Model file for the job. Use its own axes, mm. A direction names the side the tool comes from. Give positions to 0.01 mm unless a question says otherwise; leave off trailing zeros. Write each loop counter-clockwise with the first axis right and the second up, starting at its lowest first coordinate (ties: lowest second). Pieces come first, ordered by that corner, then holes.
```python
from build123d import *

# Parameters (mm, degrees)
SKETCH1_W               = 80
SKETCH1_H               = 57.5
BOSS_EXTRUDE1_DEPTH     = 8
BOSS_EXTRUDE2_START     = -10
SKETCH3_R               = 3.1
BOSS_EXTRUDE2_DEPTH     = 5
CUT_EXTRUDE1_DEPTH      = 10
CUT_EXTRUDE1_DEPTH_BACK = 63
MOVE_FACE1_BY           = 6
SKETCH5_W               = 80
SKETCH5_H               = 79.999909439
BOSS_EXTRUDE3_DEPTH     = 2
FILLET1_R               = 2
SKETCH6_R               = 2.275
CUT_EXTRUDE2_DEPTH      = 2
SKETCH7_W               = 58.936081431
SKETCH7_H               = 58.936081431
CUT_EXTRUDE3_DEPTH      = 2
FILLET2_R               = 4


with BuildPart() as part:
    # Sketch1 → Boss-Extrude1 (new body)
    with BuildSketch(Plane(origin=(0, 1.4, 0), x_dir=(1, 0, 0), z_dir=(0, 1, 0))):
        with Locations((0, 12.22)):
            Rectangle(SKETCH1_W, SKETCH1_H)
    extrude(amount=BOSS_EXTRUDE1_DEPTH)

    # Sketch3 → Boss-Extrude2 (add)
    # profile 1 of 2: a face of its own
    with BuildSketch(Plane(origin=(0, 0, -36.97), x_dir=(-1, 0, 0), z_dir=(0, 0, -1)).offset(BOSS_EXTRUDE2_START)):
        with BuildLine():
            Line((-30, 1.4), (-40, 1.4))
            Line((-40, 1.4), (-34.195661174, -6.999383953))
            ThreePointArc((-34.195661174, -6.999383953), (-26.018142719, -7.286661669), (-28.090628592, 0.629090909))
            Line((-28.090628592, 0.629090909), (-30, 1.4))
        make_face()
        with Locations(Location((-30, -4.1, 0), (0, 0, 180))):
            Circle(SKETCH3_R, mode=Mode.SUBTRACT)
    # profile 2 of 2: a face of its own
    with BuildSketch(Plane(origin=(0, 0, -36.97), x_dir=(-1, 0, 0), z_dir=(0, 0, -1)).offset(BOSS_EXTRUDE2_START)):
        with BuildLine():
            Line((34.195661174, -6.999383953), (40, 1.4))
            Line((40, 1.4), (30, 1.4))
            Line((30, 1.4), (28.090628592, 0.629090909))
            ThreePointArc((28.090628592, 0.629090909), (26.018142719, -7.286661669), (34.195661174, -6.999383953))
        make_face()
        with Locations(Location((30, -4.1, 0), (0, 0, 180))):
            Circle(SKETCH3_R, mode=Mode.SUBTRACT)
    boss_extrude2 = extrude(amount=-BOSS_EXTRUDE2_DEPTH)

    # Mirror1: Boss-Extrude2 across plane
    add(boss_extrude2.mirror(Plane.XY.offset(-13.22)))

    # Sketch4 → Cut-Extrude1 (cut, two sides: drawn at the far end of the back side and taken through both)
    with BuildSketch(Plane(origin=(0, 0, -21.97), x_dir=(-1, 0, 0), z_dir=(0, 0, -1)).offset(-CUT_EXTRUDE1_DEPTH_BACK)):
        Polygon((-30, -4.1), (-20, -9.873502692), (-40, -9.873502692), align=None)
        Polygon((20, -9.873502692), (40, -9.873502692), (30, -4.1), align=None)
    extrude(amount=CUT_EXTRUDE1_DEPTH + CUT_EXTRUDE1_DEPTH_BACK, mode=Mode.SUBTRACT)

    # Move Face1: a face moved inward by 6.0
    extrude(part.faces().sort_by_distance((0, 9.4, -12.22))[0], amount=MOVE_FACE1_BY, dir=(0, -1, 0), mode=Mode.SUBTRACT)

    # Sketch5 → Boss-Extrude3 (add)
    with BuildSketch(Plane(origin=(0, 3.4, 0), x_dir=(1, 0, 0), z_dir=(0, 1, 0))):
        with Locations((0, 23.46995472)):
            Rectangle(SKETCH5_W, SKETCH5_H)
    extrude(amount=-BOSS_EXTRUDE3_DEPTH)

    # Fillet1
    fillet1_edges = [part.edges().sort_by_distance(p)[0] for p in [
        (40, 2.4, -63.469909439),
        (-40, 2.4, -63.469909439),
        (40, 2.4, 16.53),
        (-40, 2.4, 16.53),
    ]]
    fillet(fillet1_edges, radius=FILLET1_R)

    # Sketch6 → Cut-Extrude2 (cut)
    with BuildSketch(Plane(origin=(0, 3.4, 0), x_dir=(1, 0, 0), z_dir=(0, 1, 0))):
        with Locations(Location((35.75, 59.219909439, 0), (0, 0, 180))):
            Circle(SKETCH6_R)
        with Locations(Location((35.75, -12.280045281, 0), (0, 0, 180))):
            Circle(SKETCH6_R)
        with Locations(Location((-35.74995472, 59.219909439, 0), (0, 0, 180))):
            Circle(SKETCH6_R)
        with Locations(Location((-35.74995472, -12.280045281, 0), (0, 0, 180))):
            Circle(SKETCH6_R)
    extrude(amount=-CUT_EXTRUDE2_DEPTH, mode=Mode.SUBTRACT)

    # Sketch7 → Cut-Extrude3 (cut)
    with BuildSketch(Plane(origin=(0, 3.4, 0), x_dir=(1, 0, 0), z_dir=(0, 1, 0))):
        with Locations((2.264e-05, 23.469932079)):
            Rectangle(SKETCH7_W, SKETCH7_H)
    extrude(amount=-CUT_EXTRUDE3_DEPTH, mode=Mode.SUBTRACT)

    # Fillet2
    fillet2_edges = [part.edges().sort_by_distance(p)[0] for p in [
        (29.468063356, 2.4, -52.937972794),
        (29.468063356, 2.4, 5.998108637),
        (-29.468018075, 2.4, 5.998108637),
        (-29.468018075, 2.4, -52.937972794),
    ]]
    fillet(fillet2_edges, radius=FILLET2_R)


solid = part.part
```
1. Which spindle directions (+Z, -Z, +X, -X, +Y, -Y) get a long thin tool onto all of the face, cutting with end or side? Do faces 5 (the flat face through (33, -2, -26.97)), 6 (the flat face through (-26.461, -6.143, -1.935)), 7 (the flat face through (33, -2, 0.53)), 8 (the cylindrical face through (25.159, -2.497, -24.505)). Say none if no direction does.
Calculated:
face 5: -Z, +X, -X, -Y
face 6: +Z, -Z, -Y
face 7: +Z, +X, -X, -Y
face 8: +Z, -Z
2. Slice it at C-C, the plane y = -2.25. State how many separate pieces and enclosed holes the cut face has, and give its area (3 significant figures).
Calculated:
separate pieces: 8
enclosed holes: 0
area: 145 mm2
3. Probe probe 1 along Z at (x, y) = (35.75, 2.55); probe 2 along X at (y, z) = (2.75, -59.5); probe 3 along X at (y, z) = (1.5, 2). List the from-to ranges inside material, lowest first.
Calculated:
probe 1: z = -63.47 to -61.49, -56.94 to 10.01, 14.56 to 16.53
probe 2: x = -40 to -38.01, -33.49 to 33.49, 38.01 to 40
probe 3: x = -40 to -29.47, 29.47 to 40
4. Slice it at B-B, the plane x = -4. Write the cut outline in (y, z).
Calculated:
outline: (1.4, -63.47) - (3.4, -63.47) - (3.4, -52.94) - (1.4, -52.94) - close; (1.4, 6) - (3.4, 6) - (3.4, 16.53) - (1.4, 16.53) - close
5. Slice it at D-D, the plane x = 35.75. Write the cut outline in (y, z), and give its area (3 significant figures).
Calculated:
outline: (-4.75, -26.97) - (1.4, -26.97) - (1.4, -56.94) - (3.4, -56.94) - (3.4, 10.01) - (1.4, 10.01) - (1.4, 0.53) - (-4.75, 0.53) - (-4.75, -4.47) - (1.4, -4.47) - (1.4, -21.97) - (-4.75, -21.97) - close; (1.4, -63.47) - (3.4, -63.47) - (3.4, -61.49) - (1.4, -61.49) - close; (1.4, 14.56) - (3.4, 14.56) - (3.4, 16.53) - (1.4, 16.53) - close
area: 203 mm2
6. Pin check, flat tips, straight feed: P1, Ø4, axis at x = 8, y = -1.5, coming from the +Z side; P2, Ø2.5, axis at x = 31, y = -1.5, coming from the +Z side; P3, Ø6, axis at x = -35.75, z = -59.22, coming from the -Y side; P4, Ø6, axis at x = -35.75, z = 12.28, coming from the +Y side. Stop position of each tip, or through.
Calculated:
P1: passes through
P2: stops at z = 0.53
P3: stops at y = 1.4
P4: stops at y = 3.4
7. Pull direction X, two halves, no side cores. Call faces 1 (the cylindrical face through (39.43, 2.41, 15.93)), 2 (the cylindrical face through (-25.2, -2.38, -1.94)), 3 (the cylindrical face through (-30, -1, -2)), 4 (the flat face through (-37.177, -2.686, -24.505)): +X half, -X half, draft (parallel to the pull), parting line (faces both ways), or undercut.
Calculated:
face 1: +X half
face 2: undercut
face 3: undercut
face 4: -X half
8. Slice it at A-A, the plane z = -30. Write the cut outline in (x, y), and give its area (3 significant figures).
Calculated:
outline: (-40, 1.4) - (-29.47, 1.4) - (-29.47, 3.4) - (-40, 3.4) - close; (29.47, 1.4) - (40, 1.4) - (40, 3.4) - (29.47, 3.4) - close
area: 42.1 mm2
